Part model, mm, in its own coordinate system. Coordinates: 2 decimals unless noted, no trailing zeros. Loops run counter-clockwise (first coordinate to the right, second up) from the corner with the lowest first, then second, coordinate; pieces in that order, holes last. Notation, with made-up numbers: (21, 14.25) - (58, 14.25) arc R8 ccw to (58, 22.25) - close; hole circle Ø6 at (9, -19.5). An arc over 180 degrees is marked (long way). Answer as CSV lines item,"result".
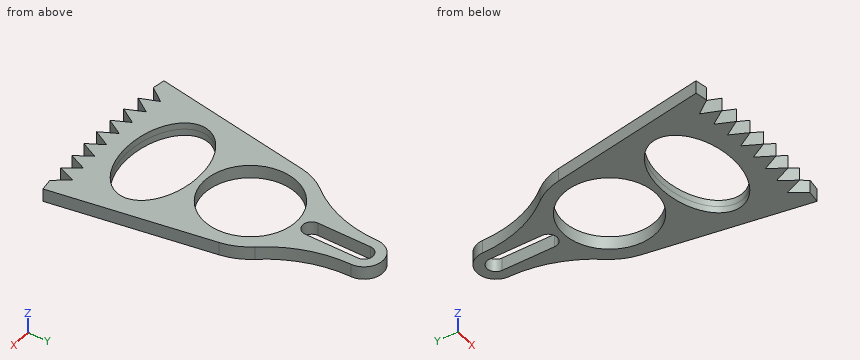
from build123d import *

# Parameters (mm, degrees)
SKETCH1_R           = 7
SKETCH1_RX          = 8.5
SKETCH1_RY          = 5.35
BOSS_EXTRUDE1_DEPTH = 1
CUT_EXTRUDE1_DEPTH  = 27.930466019


with BuildPart() as part:
    # Sketch1 → Boss-Extrude1 (new, symmetric)
    with BuildSketch(Plane.XY):
        with BuildLine():
            Line((-13, -22.436683487), (-8.869214361, 1.528736933))
            ThreePointArc((-8.869214361, 1.528736933), (-8.195662334, 3.719021229), (-6.990807006, 5.668211129))
            ThreePointArc((-6.990807006, 5.668211129), (-3.915823856, 11.153015373), (-2.85, 17.35))
            ThreePointArc((-2.85, 17.35), (0, 20.2), (2.85, 17.35))
            ThreePointArc((2.85, 17.35), (3.915823856, 11.153015373), (6.990807006, 5.668211129))
            ThreePointArc((6.990807006, 5.668211129), (8.195662334, 3.719021229), (8.869214361, 1.528736933))
            Line((8.869214361, 1.528736933), (13, -22.436683487))
            ThreePointArc((13, -22.436683487), (0, -23.5), (-13, -22.436683487))
        make_face()
        Circle(SKETCH1_R, mode=Mode.SUBTRACT)
        with Locations(Location((0, -13.35), (0, 0, 180))):
            Ellipse(SKETCH1_RX, SKETCH1_RY, mode=Mode.SUBTRACT)
        with BuildLine():
            Line((-1.35, 9.35), (-1.35, 17.35))
            ThreePointArc((-1.35, 17.35), (0, 18.7), (1.35, 17.35))
            Line((1.35, 17.35), (1.35, 9.35))
            ThreePointArc((1.35, 9.35), (0, 8), (-1.35, 9.35))
        make_face(mode=Mode.SUBTRACT)
    extrude(amount=BOSS_EXTRUDE1_DEPTH, both=True)

    # Sketch2 → Cut-Extrude1 (cut, through all)
    with BuildSketch(Plane.XY.offset(1)):
        with BuildLine():
            ThreePointArc((-11.133848077, -22.721445499), (-9.749547472, -22.903692131), (-8.362277061, -23.061751629))
            Line((-8.362277061, -23.061751629), (-9.444827704, -20.421948771))
            Line((-9.444827704, -20.421948771), (-11.133848077, -22.721445499))
        make_face()
        with BuildLine():
            ThreePointArc((-8.362277061, -23.061751629), (-6.97245942, -23.195575847), (-5.5805179, -23.305124021))
            Line((-5.5805179, -23.305124021), (-6.754536872, -20.704709731))
            Line((-6.754536872, -20.704709731), (-8.362277061, -23.061751629))
        make_face()
        with BuildLine():
            ThreePointArc((-5.5805179, -23.305124021), (-4.186876499, -23.39036278), (-2.791959736, -23.451266162))
            Line((-2.791959736, -23.451266162), (-4.056016678, -20.893408645))
            Line((-4.056016678, -20.893408645), (-5.5805179, -23.305124021))
        make_face()
        with BuildLine():
            Line((-1.352554853, -20.987815613), (-2.791959736, -23.451266162))
            ThreePointArc((-2.791959736, -23.451266162), (-1.396192515, -23.487815613), (0, -23.5))
            Line((0, -23.5), (-1.352554853, -20.987815613))
        make_face()
    cut_extrude1 = extrude(amount=-CUT_EXTRUDE1_DEPTH, mode=Mode.SUBTRACT)

    # Mirror1: Cut-Extrude1 across plane
    add(cut_extrude1.mirror(Plane(origin=(0, 0, 0), x_dir=(0, 0, 1), z_dir=(1, 0, 0))), mode=Mode.SUBTRACT)


solid = part.part
Q1. Saw through at A-A (y = 3). Give the cut face in (x, z), then the cut area to 3 significant figures.
Results:
outline,"(-8.49, -1) - (-6.32, -1) - (-6.32, 1) - (-8.49, 1) - close; (6.32, -1) - (8.49, -1) - (8.49, 1) - (6.32, 1) - close"
area,"8.64 mm^2"
Q2. Flat gauge pins, fed straight in: pin 1 (0.6 mm diameter, centred on y = 13.5, z = -0.5, fed in from +X); pin 2 (1 mm diameter, centred on y = 14.5, z = -0.5, fed in from -X) (3 decimals). Where does each tip first touch, or does it go through?
Results:
pin 1,"stops at x = 3.32"
pin 2,"stops at x = -3.155"
Q3. Wall check: L1, parallel to X at y = 17, z = -0.3; L2, parallel to Y at x = -1.5, z = -0.8; L3, parallel to Y at x = -2.5, z = 0.1. Give the ranges that are in metal, low to high.
Results:
L1,"x = -2.85 to -1.35, 1.35 to 2.85"
L2,"y = -21.24 to -18.62, -8.08 to -6.84, 6.84 to 19.77"
L3,"y = -22.95 to -18.46, -8.24 to -6.54, 6.54 to 18.72"
Q4. Saw through at B-B (z = -0.6). Count the separate pieces of the cut face and the enclosed holes in it, then the cut area to 3 significant figures.
Results:
separate pieces,"1"
enclosed holes,"3"
area,"368 mm^2"
